```python
from build123d import *

# Parameters (mm, degrees)
SKETCH1_R           = 2.032
BOSS_EXTRUDE1_DEPTH = 9.525
SKETCH2_R           = 2.032
CUT_EXTRUDE1_DEPTH  = 29.925626614
FILLET1_R           = 1.5875


with BuildPart() as part:
    # Sketch1 → Boss-Extrude1 (new body)
    with BuildSketch(Plane.XY):
        with BuildLine():
            Line((0, 0), (0, 5.08))
            ThreePointArc((0, 5.08), (0.227086506, 6.259165397), (0.875862069, 7.269655172))
            Line((0.875862069, 7.269655172), (7.663793103, 14.396982759))
            ThreePointArc((7.663793103, 14.396982759), (11.1125, 15.875), (14.561206897, 14.396982759))
            Line((14.561206897, 14.396982759), (21.349137931, 7.269655172))
            ThreePointArc((21.349137931, 7.269655172), (21.997913494, 6.259165397), (22.225, 5.08))
            Line((22.225, 5.08), (22.225, 0))
            Line((22.225, 0), (0, 0))
        make_face()
        with Locations(Location((11.1125, 11.1125, 0), (0, 0, 180))):
            Circle(SKETCH1_R, mode=Mode.SUBTRACT)
    extrude(amount=BOSS_EXTRUDE1_DEPTH)

    # Sketch2 → Cut-Extrude1 (cut, through all)
    with BuildSketch(Plane.XZ):
        with Locations(Location((4.7625, 4.7625, 0), (0, 0, 270))):
            Circle(SKETCH2_R)
        with Locations(Location((17.4625, 4.7625, 0), (0, 0, 270))):
            Circle(SKETCH2_R)
    extrude(amount=-CUT_EXTRUDE1_DEPTH, mode=Mode.SUBTRACT)

    # Fillet1
    fillet1_edges = [part.edges().sort_by_distance(p)[0] for p in [
        (17.955172414, 10.833318966, 0),
        (21.997913494, 6.259165397, 0),
        (22.225, 2.54, 0),
        (21.997913494, 6.259165397, 9.525),
        (17.955172414, 10.833318966, 9.525),
        (11.1125, 15.875, 9.525),
        (4.269827586, 10.833318966, 9.525),
        (0.227086506, 6.259165397, 9.525),
        (0, 2.54, 9.525),
        (0, 2.54, 0),
        (22.225, 2.54, 9.525),
        (0.227086506, 6.259165397, 0),
        (4.269827586, 10.833318966, 0),
        (11.1125, 15.875, 0),
    ]]
    fillet(fillet1_edges, radius=FILLET1_R)


solid = part.part
```
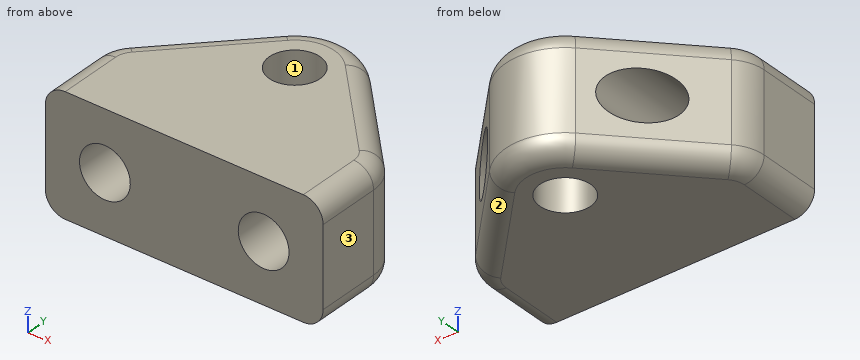
Model file for the job. Use its own axes, mm. Face numbers are marked on the shaded views. Give positions to 0.01 mm unless a question says otherwise; leave off trailing zeros. Loops run counter-clockwise (first coordinate to the right, second up) from the corner with the lowest first, then second, coordinate; pieces in that order, holes last. Notation, with made-up numbers: M 74,38.25 L 132,38.25 A28 cw 132,57.25 Z; hole C -39.5,60 d11. An arc over 180 degrees is marked long. Use one line per item in the form item = value.
Item 1: Flat gauge pins, fed straight in: pin 1 Ø5.5 at (x, z) = (17.46, 4.76) entering from +Y; pin 2 Ø2 at (x, z) = (19.5, 5) entering from +Y; pin 3 Ø1 at (x, y) = (3, 8.5) entering from -Z. Where does each tip first touch, or does it go through?
Filled in:
pin_1 = 14.24
pin_2 = 9.6
pin_3 = 0.05
Item 2: Two-plate mould, pull along Y, no slides. Class the marked faces 1, 2 and 3: released by +Y, released by -Y, zero draft, split by the parting line, or undercut.
Filled in:
face_1 = undercut
face_2 = released by +Y
face_3 = zero draft
Item 3: Slice it at C-C on y = 1. List the corners of the cut face in (x, z) (1 decimal), and give its area (3 significant figures).
Filled in:
outline = M 0,1.6 A1.6 ccw 1.6,0 L 20.6,0 A1.6 ccw 22.2,1.6 L 22.2,7.9 A1.6 ccw 20.6,9.5 L 1.6,9.5 A1.6 ccw 0,7.9 Z; hole C 4.8,4.8 d4.1; hole C 17.5,4.8 d4.1
area = 184 mm^2
Item 4: Slice it at A-A on z = 4.75. Give the number of separate pieces and of enclosed holes in the cut face, and give its area (3 significant figures).
Filled in:
separate_pieces = 3
enclosed_holes = 1
area = 160 mm^2
Item 5: Drill centre lines: L1, parallel to X at y = 0.5, z = 5.75 (3 decimals); L2, parallel to Y at x = 11.25, z = 4.5; L3, parallel to Z at x = 3.25, y = 4 (3 decimals). Where is each one in solid material? Low to high.
Filled in:
L1 = 0 to 2.987, 6.538 to 15.687, 19.238 to 22.225
L2 = 0 to 9.09, 13.14 to 15.87
L3 = 0 to 3.406, 6.119 to 9.525
